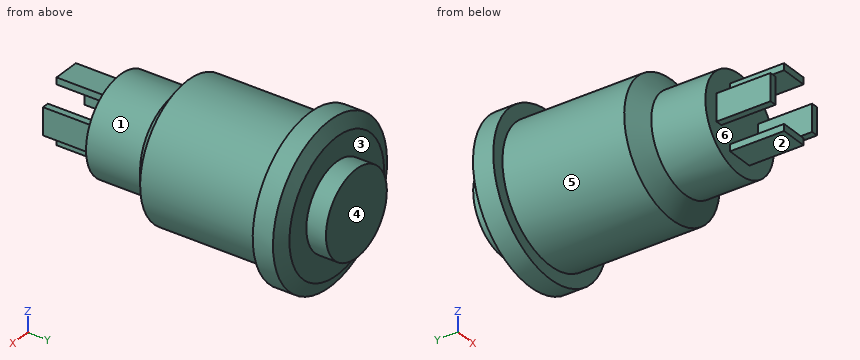
from build123d import *

# Parameters (mm, degrees)
ESQUISSE2_W                  = 2
ESQUISSE2_H                  = 0.5
BOSS_EXTRU_1_DEPTH           = 4
R_P_TITION_CIRCULAIRE1_COUNT = 4


with BuildPart() as part:
    # Esquisse1 → Révolution1 (revolve)
    with BuildSketch(Plane.XY, mode=Mode.PRIVATE) as r_volution1_sk:
        Polygon((0, 3.45), (-3.15, 3.45), (-3.15, 2), (-4.9, 2), (-5.9, 1.5), (-5.9, 0), (-4.95, 0), (-4.95, -9), (-3.55, -10), (-3.55, -14), (0, -14), align=None)
    revolve(r_volution1_sk.sketch.rotate(Axis((0, 55, 0), (0, -1, 0)), 270), axis=Axis((0, 55, 0), (0, -1, 0)))

    # Esquisse2 → Boss.-Extru.1 (add)
    with BuildSketch(Plane.XZ.offset(14)):
        with Locations((0, 2.15)):
            Rectangle(ESQUISSE2_W, ESQUISSE2_H)
    boss_extru_1 = extrude(amount=BOSS_EXTRU_1_DEPTH)

    # Répétition circulaire1: Boss.-Extru.1 ×4 about axis
    r_p_tition_circulaire1_axis = Axis((0, 0, 0), (0, 1, 0))
    for i in range(1, R_P_TITION_CIRCULAIRE1_COUNT):
        add(boss_extru_1.rotate(r_p_tition_circulaire1_axis, i * 360 / R_P_TITION_CIRCULAIRE1_COUNT))


solid = part.part
The listing builds one solid part. Answer for the finished solid, in the listing's coordinates (mm). Face numbers are marked on the shaded views. A direction names the side the tool comes from. Coordinates: 2 decimals unless noted, no trailing zeros. Write each loop counter-clockwise with the first axis right and the second up, starting at its lowest first coordinate (ties: lowest second). Pieces come first, ordered by that corner, then holes. Notation, with made-up numbers: M 8,59.5 L 43,59.5 A21 cw 43,81.5 Z; hole C -0.5,66.5 d7. An arc over 180 degrees is marked long. Write each question's results on one line, items separated by ' | '.
Item 1: The part is cut by section C-C on z = 0. Determine the outline of the cut face in (x, y).
Answer below:
outline: M -5.9,0 L -4.95,0 L -4.95,-9 L -3.55,-10 L -3.55,-14 L -2.4,-14 L -2.4,-18 L -1.9,-18 L -1.9,-14 L 1.9,-14 L 1.9,-18 L 2.4,-18 L 2.4,-14 L 3.55,-14 L 3.55,-10 L 4.95,-9 L 4.95,0 L 5.9,0 L 5.9,1.5 L 4.9,2 L 3.15,2 L 3.15,3.45 L -3.15,3.45 L -3.15,2 L -4.9,2 L -5.9,1.5 Z
Item 2: The part is cut by section D-D on y = -1.5. Determine the outline of the cut face in (x, z), and give its area (3 significant figures).
Answer below:
outline: C 0,0 d9.9 | area: 77.0 mm2
Item 3: The part is cut by section A-A on y = -14.5. Determine the outline of the cut face in (x, z), and give its area (3 significant figures).
Answer below:
outline: M -2.4,-1 L -1.9,-1 L -1.9,1 L -2.4,1 Z; M -1,-2.4 L 1,-2.4 L 1,-1.9 L -1,-1.9 Z; M -1,1.9 L 1,1.9 L 1,2.4 L -1,2.4 Z; M 1.9,-1 L 2.4,-1 L 2.4,1 L 1.9,1 Z | area: 4.00 mm2
Item 4: Consider probe 1 along Y at (x, z) = (-1, -1.5); probe 2 along Y at (x, z) = (-3, -1.25); probe 3 along X at (y, z) = (-5.75, -2). Determine where each line is inside the solid, lowest interval first. Write a range as [from, to].
Answer below:
probe 1: [-14, 3.45] | probe 2: [-14, 2] | probe 3: [-4.53, 4.53]
Item 5: For a pull along X with two mould halves and no side action, classify the marked faces 4, 5 and 6 as released by +X, released by -X, zero draft, split by the parting line, or undercut.
Answer below:
face 4: zero draft | face 5: split by the parting line | face 6: undercut
Item 6: The part is cut by section B-B on x = 0. Determine the outline of the cut face in (y, z).
Answer below:
outline: M -18,-2.4 L -14,-2.4 L -14,-3.55 L -10,-3.55 L -9,-4.95 L 0,-4.95 L 0,-5.9 L 1.5,-5.9 L 2,-4.9 L 2,-3.15 L 3.45,-3.15 L 3.45,3.15 L 2,3.15 L 2,4.9 L 1.5,5.9 L 0,5.9 L 0,4.95 L -9,4.95 L -10,3.55 L -14,3.55 L -14,2.4 L -18,2.4 L -18,1.9 L -14,1.9 L -14,-1.9 L -18,-1.9 Z
Item 7: Given P1, Ø1.5, axis at x = 2, y = -12, coming from the +Z side; P2, Ø2, axis at x = -0.5, z = 0, coming from the -Y side; P3, Ø2, axis at y = -5, z = -4, coming from the +X side, each flat-ended and moving along its own axis, determine where each tip first touches the part or whether it passes through.
Answer below:
P1: z = 3.32 | P2: y = -14 | P3: x = 3.94
Item 8: Which of the six approach directions +Z, -Z, +X, -X, +Y, -Y give full straight-line access (tool end or side, diameter ignored) to the marked faces 1, 2 and 3?
Answer below:
face 1: -Y | face 2: -Z, +X, -X, -Y | face 3: +Y
